```python
from build123d import *

# Parameters (mm, degrees)
BOSS_EXTRUDE1_DEPTH = 241.3
BOSS_EXTRUDE1_DRAFT = -5
SHELL1_T            = -19.05


with BuildPart() as part:
    # Sketch1 → Boss-Extrude1 (with draft: the straight prism first)
    with BuildSketch(Plane(origin=(0, 0, 0), x_dir=(1, 0, 0), z_dir=(0, 1, 0))):
        Polygon((122.672579939, 0), (106.237570575, 61.336289969), (61.336289969, 106.237570575), (0, 122.672579939), (-61.336289969, 106.237570575), (-106.237570575, 61.336289969), (-122.672579939, 0), (-106.237570575, -61.336289969), (-61.336289969, -106.237570575), (0, -122.672579939), (61.336289969, -106.237570575), (106.237570575, -61.336289969), align=None)
    extrude(amount=-BOSS_EXTRUDE1_DEPTH)
    # Boss-Extrude1: the draft: its side faces are tilted about the plane it starts from
    boss_extrude1_sides = [part.faces().sort_by_distance(p)[0] for p in [
        (114.455075257, -120.65, -30.668144985),
        (83.786930272, -120.65, -83.786930272),
        (30.668144985, -120.65, -114.455075257),
        (-30.668144985, -120.65, -114.455075257),
        (-83.786930272, -120.65, -83.786930272),
        (-114.455075257, -120.65, -30.668144985),
        (-114.455075257, -120.65, 30.668144985),
        (-83.786930272, -120.65, 83.786930272),
        (-30.668144985, -120.65, 114.455075257),
        (30.668144985, -120.65, 114.455075257),
        (83.786930272, -120.65, 83.786930272),
        (114.455075257, -120.65, 30.668144985),
    ]]
    draft(boss_extrude1_sides, Plane(origin=(0, 0, 0), x_dir=(1, 0, 0), z_dir=(0, 1, 0)), BOSS_EXTRUDE1_DRAFT)

    # Shell1
    shell1_openings = [part.faces().sort_by_distance(p)[0] for p in [
        (0, -241.3, 0),
        (0, 0, 0),
    ]]
    offset(amount=SHELL1_T, openings=shell1_openings, kind=Kind.INTERSECTION)


solid = part.part
```
Can you work these out from the model? Positions are in its coordinate system, mm. A direction names the side the tool comes from. Round coordinates to 2 decimals unless told otherwise and drop trailing zeros. Loops run counter-clockwise (first coordinate to the right, second up) from the corner with the lowest first, then second, coordinate; pieces in that order, holes last.
Item 1: Suppose I cut it at B-B, the plane y = -80.5. Write out the boundary of the cut face in (x, z), then the cut area to 3 significant figures.
Item 2: Which directions (+Z, -Z, +X, -X, +Y, -Y) give clear straight access to the entire face, cutting with the end or side of a thin tool? Please do faces 1 (the flat face through (-104.29, -118.96, -28.4)), 2 (the flat face through (62.64, -118.96, 63.17)).
Item 3: Please list where these lines run through material, in increasing order: L1, parallel to Z at x = -18.5, y = -98.5; L2, parallel to X at y = -65, z = 65.5; L3, parallel to Z at x = -68, y = -69.
Item 4: Suppose I cut it at A-A, the plane x = 75. Write out the boundary of the cut face in (y, z).
Item 5: Will these pins go through, and if not, where does the flat tip stop? pin 1 Ø6 at (x, y) = (92, -209) entering from +Z; pin 2 Ø6 at (x, y) = (30.5, -187) entering from -Z; pin 3 Ø10 at (x, y) = (12, -120) entering from +Z.
Item 6: Suppose I cut it at C-C, the plane z = -10. Write out the boundary of the cut face in (x, y).
Item 7: If we mould it in two halves opening along Z, with no side actions, what happens to faces 3 (the flat face through (-63.17, -118.96, 62.64)), 4 (the flat face through (-27.545, -118.961, -104.517)), 5 (the flat face through (-60, -241.3, 52)), 6 (the flat face through (27.545, -118.961, 104.517))? For each: +Z half, -Z half, draft (parallel to the pull), parting line (faces both ways), or undercut.
Item 8: Suppose I cut it at D-D, the plane x = 18. Write out the boundary of the cut face in (y, z), then the cut area to 3 significant figures.
Reported:
1. outline: (-115.38, 0) - (-99.92, -57.69) - (-57.69, -99.92) - (0, -115.38) - (57.69, -99.92) - (99.92, -57.69) - (115.38, 0) - (99.92, 57.69) - (57.69, 99.92) - (0, 115.38) - (-57.69, 99.92) - (-99.92, 57.69) - close; hole (-95.58, 0) - (-82.78, -47.79) - (-47.79, -82.78) - (0, -95.58) - (47.79, -82.78) - (82.78, -47.79) - (95.58, 0) - (82.78, 47.79) - (47.79, 82.78) - (0, 95.58) - (-47.79, 82.78) - (-82.78, 47.79) - close
1. area: 12,500 mm2
2. face 1: -Z, -X, -Y
2. face 2: +Y
3. L1: z = -108.79 to -89, 89 to 108.79
3. L2: x = -94.03 to -66.99, 66.99 to 94.03
3. L3: z = -91.04 to -63.99, 63.99 to 91.04
4. outline: (-241.3, -62.72) - (0, -92.57) - (0, -65.53) - (-179.66, -43.3) - (-241.3, -22.47) - close; (-241.3, 22.47) - (-179.66, 43.3) - (0, 65.53) - (0, 92.57) - (-241.3, 62.72) - close
5. pin 1: stops at z = 52.74
5. pin 2: stops at z = -98.41
5. pin 3: stops at z = 110
6. outline: (-119.99, 0) - (-98.14, -241.3) - (-78.34, -241.3) - (-100.2, 0) - close; (78.34, -241.3) - (98.14, -241.3) - (119.99, 0) - (100.2, 0) - close
7. face 3: undercut
7. face 4: -Z half
7. face 5: draft
7. face 6: +Z half
8. outline: (-241.3, -95.99) - (0, -117.85) - (0, -98.05) - (-241.3, -76.2) - close; (-241.3, 76.2) - (0, 98.05) - (0, 117.85) - (-241.3, 95.99) - close
8. area: 9,550 mm2
